Here's the drawing with two shaded views (mm, measured from the low corner). I have some questions. Coordinates: 2 decimals unless noted, no trailing zeros. Order: outer loops, then holes, each group sorted by start corner. A loop starts at its lowest first (then second) coordinate and runs counter-clockwise, first axis right, second up. Notation, with made-up numbers: (37, 85) - (85, 85) arc R13 ccw to (85, 90) - close; hole circle Ø9 at (59, -8). An arc over 180 degrees is marked (long way). Answer as a JSON object with one key per item and string values. Group by question number.
(1) Imagine slicing it at B-B, the plane z = 11.5. Write out the boundary of the cut face in (x, y) (3 decimals).
(2) Please list where these lines run through material, in increasing order: probe 1 along X at (y, z) = (5, 10.5); probe 2 along Y at (x, z) = (19, 4); probe 3 along X at (y, z) = (20.5, 0.9) (3 decimals).
(3) Imagine slicing it at C-C, the plane y = 32. Write out the boundary of the cut face in (x, z).
(4) Imagine slicing it at D-D, the plane x = 17. Write out the boundary of the cut face in (y, z), and give its area (3 significant figures).
(5) Imagine slicing it at A-A, the plane y = 20.5. Write out the boundary of the cut face in (x, z) (3 decimals).
(6) We'd pull the mould along X, two halves only. Please class the marked faces 1, 2, 3 and 4: pulls with the +X half, pulls with the -X half, needs draft (parallel to the pull), parting line crosses it, or undercut.
(7) Will these pins go through, and if not, where does the flat tip stop? P1, Ø1.6, axis at y = 15.5, z = 10, coming from the +X side; P2, Ø6, axis at y = 28, z = 5.5, coming from the -X side; P3, Ø1, axis at y = 32, z = 8.5, coming from the -X side.
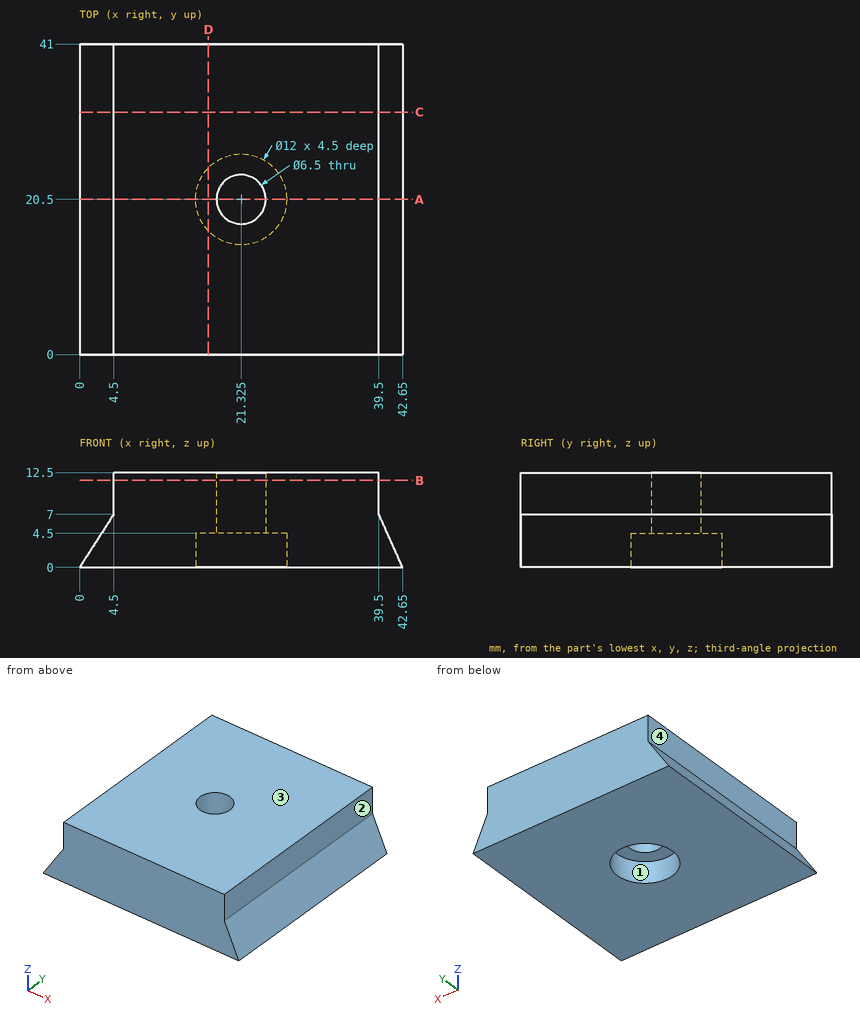
Result set:
{
 "1": {"outline": "(4.5, 0) - (39.5, 0) - (39.5, 41) - (4.5, 41) - close; hole circle Ø6.5 at (21.325, 20.5)"},
 "2": {"probe 1": "x = 4.5 to 39.5", "probe 2": "y = 0 to 14.97, 26.03 to 41", "probe 3": "x = 0.579 to 15.325, 27.325 to 42.245"},
 "3": {"outline": "(0, 0) - (42.65, 0) - (39.5, 7) - (39.5, 12.5) - (4.5, 12.5) - (4.5, 7) - close"},
 "4": {"outline": "(0, 0) - (16.34, 0) - (16.34, 4.5) - (24.66, 4.5) - (24.66, 0) - (41, 0) - (41, 12.5) - (0, 12.5) - close", "area": "475 mm^2"},
 "5": {"outline": "(0, 0) - (15.325, 0) - (15.325, 4.5) - (18.075, 4.5) - (18.075, 12.5) - (4.5, 12.5) - (4.5, 7) - close; (24.575, 4.5) - (27.325, 4.5) - (27.325, 0) - (42.65, 0) - (39.5, 7) - (39.5, 12.5) - (24.575, 12.5) - close"},
 "6": {"face 1": "undercut", "face 2": "pulls with the +X half", "face 3": "needs draft", "face 4": "pulls with the -X half"},
 "7": {"P1": "stops at x = 39.5", "P2": "stops at x = 1.61", "P3": "stops at x = 4.5"}
}
